Could you check a few things on this model? Use its own coordinates, in mm. Face numbers are marked on the shaded views. A direction names the side the tool comes from. Coordinates: 2 decimals unless noted, no trailing zeros. Order: outer loops, then holes, each group sorted by start corner. A loop starts at its lowest first (then second) coordinate and runs counter-clockwise, first axis right, second up. Notation, with made-up numbers: (32, 24.25) - (65, 24.25) arc R27 ccw to (65, 43.25) - close; hole circle Ø10 at (89, 61.5). An arc over 180 degrees is marked (long way). Answer as a JSON object with one key per item and string values. Group by question number.
(1) Imagine slicing it at C-C, the plane z = 6.5. Write out the boundary of the cut face in (x, y) (1 decimal).
(2) Which directions (+Z, -Z, +X, -X, +Y, -Y) give clear straight access to the entire face, cutting with the end or side of a thin tool? Please do the marked faces 1 and 2.
(3) Will these pins go through, and if not, where does the flat tip stop? P1, Ø3, axis at x = 1, z = 10.5, coming from the -Y side; P2, Ø12.5, axis at x = 3, z = 3.5, coming from the -Y side; P3, Ø5, axis at x = 13.5, z = 6, coming from the -Y side; P4, Ø2, axis at y = -23, z = 1.5, coming from the +X side.
(4) We'd pull the mould along Y, two halves only. Please class the marked faces 3, 4, 5 and 6: pulls with the +Y half, pulls with the -Y half, needs draft (parallel to the pull), parting line crosses it, or undercut.
(5) Please list where these lines run through material, in increasing order: probe 1 along X at (y, z) = (-20, -0.5); probe 2 along Y at (x, z) = (5, -3); probe 3 along Z at (x, y) = (15.5, -20).
(6) Imagine slicing it at B-B, the plane y = -28.5. Write out the boundary of the cut face in (x, z).
(7) Imagine slicing it at A-A, the plane y = -19.5. Write out the boundary of the cut face in (x, z).
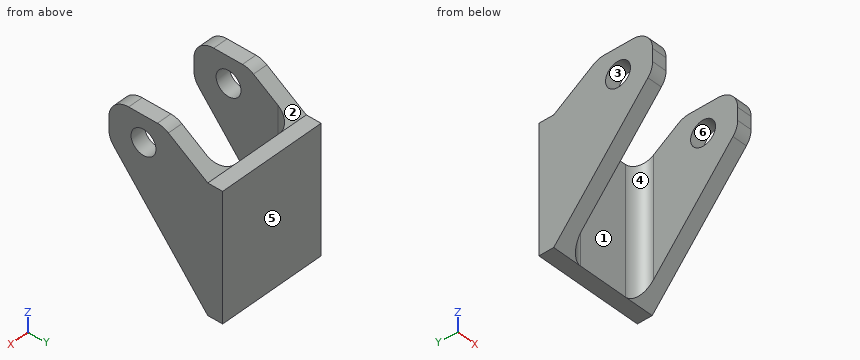
from build123d import *

# Parameters (mm, degrees)
SKETCH1_W           = 4.7625
SKETCH1_H           = 50
SKETCH1_W_2         = 25.4
BOSS_EXTRUDE1_DEPTH = 4.7625
SKETCH1_3_W         = 4.7625
SKETCH1_3_H         = 50
BOSS_EXTRUDE2_DEPTH = 31.75
SKETCH3_R           = 4
CUT_EXTRUDE1_DEPTH  = 35.925
FILLET1_R           = 6.35
FILLET2_R           = 4.7625


with BuildPart() as part:
    # Sketch1 → Boss-Extrude1 (new body)
    with BuildSketch(Plane(origin=(0, 0, 0), x_dir=(1, 0, 0), z_dir=(0, 1, 0))):
        with Locations((-15.08125, 0)):
            Rectangle(SKETCH1_W, SKETCH1_H)
        Rectangle(SKETCH1_W_2, SKETCH1_H)
        with Locations((15.08125, 0)):
            Rectangle(SKETCH1_W, SKETCH1_H)
    extrude(amount=BOSS_EXTRUDE1_DEPTH)

    # Sketch1<3> → Boss-Extrude2 (add)
    with BuildSketch(Plane(origin=(0, 0, 0), x_dir=(1, 0, 0), z_dir=(0, 1, 0))):
        with Locations((-15.08125, 0)):
            Rectangle(SKETCH1_3_W, SKETCH1_3_H)
        with Locations((15.08125, 0)):
            Rectangle(SKETCH1_3_W, SKETCH1_3_H)
    extrude(amount=-BOSS_EXTRUDE2_DEPTH)

    # Sketch3 → Cut-Extrude1 (cut, through all)
    with BuildSketch(Plane(origin=(17.4625, 0, 0), x_dir=(0, 0, -1), z_dir=(1, 0, 0))):
        Polygon((25, -31.75), (25, 0), (-12.3, -31.75), align=None)
        Polygon((-15.475, 0), (-15.475, 4.7625), (-25, 4.7625), (-25, 0), (-25, -14.247596398), align=None)
        with Locations((-16.745, -20.6375)):
            Circle(SKETCH3_R)
    extrude(amount=-CUT_EXTRUDE1_DEPTH, mode=Mode.SUBTRACT)

    # Fillet1
    fillet1_edges = [part.edges().sort_by_distance(p)[0] for p in [
        (-15.08125, -31.75, 25),
        (15.08125, -31.75, 25),
        (15.08125, -31.75, 12.3),
        (-15.08125, -31.75, 12.3),
        (15.08125, -14.247596398, 25),
        (-15.08125, -14.247596398, 25),
    ]]
    fillet(fillet1_edges, radius=FILLET1_R)

    # Fillet2
    fillet2_edges = [part.edges().sort_by_distance(p)[0] for p in [
        (12.7, 0, -4.7625),
        (-12.7, 0, -4.7625),
    ]]
    fillet(fillet2_edges, radius=FILLET2_R)


solid = part.part
Result set:
{
 "1": {"outline": "(-17.5, -26.8) - (-12.7, -26.8) - (-12.7, -4.8) arc R4.8 cw to (-7.9, 0) - (7.9, 0) arc R4.8 cw to (12.7, -4.8) - (12.7, -26.8) - (17.5, -26.8) - (17.5, 4.8) - (-17.5, 4.8) - close"},
 "2": {"face 1": "+Z, -Z, -Y", "face 2": "+Z, +X, -X, +Y"},
 "3": {"P1": "stops at y = 0", "P2": "stops at y = -0.18", "P3": "stops at y = -28.52", "P4": "stops at x = 17.46"},
 "4": {"face 3": "undercut", "face 4": "pulls with the -Y half", "face 5": "pulls with the +Y half", "face 6": "undercut"},
 "5": {"probe 1": "x = -17.46 to -12.7, 12.7 to 17.46", "probe 2": "y = 0 to 4.76", "probe 3": "z = -1.5 to 12.8, 20.69 to 25"},
 "6": {"outline": "(-17.46, 8.48) - (-12.7, 8.48) - (-12.7, 24.19) - (-17.46, 24.19) - close; (12.7, 8.48) - (17.46, 8.48) - (17.46, 24.19) - (12.7, 24.19) - close"},
 "7": {"outline": "(-17.46, -2.09) - (-12.7, -2.09) - (-12.7, 12.91) - (-17.46, 12.91) - close; (-17.46, 20.58) - (-12.7, 20.58) - (-12.7, 25) - (-17.46, 25) - close; (12.7, -2.09) - (17.46, -2.09) - (17.46, 12.91) - (12.7, 12.91) - close; (12.7, 20.58) - (17.46, 20.58) - (17.46, 25) - (12.7, 25) - close"}
}
